Autodesk Inventor part; units mm, degrees
ref_plane "YZ Plane" through (0, 0, 0) normal (1, 0, 0) x (0, 1, 0)
ref_plane "XZ Plane" through (0, 0, 0) normal (0, 1, 0) x (-1, 0, 0)
ref_plane "XY Plane" through (0, 0, 0) normal (0, 0, 1) x (1, 0, 0)
sketch "Sketch1" plane through (0, 0, 0) normal (0, 1, 0) x (-1, 0, 0)
  line L0 (0, 0) -> (29.7942, 0)
  line L1 (29.7942, 0) -> (29.7942, -38.1)
  line L2 (29.7942, -38.1) -> (0, -38.1)
  line L3 (0, -38.1) -> (0, 0)
  circle A0 centre (21.844, -9.525) radius 1.905
  circle A1 centre (8.255, -29.845) radius 1.905
  dimension "d0" = 29.7942
  dimension "d1" = 38.1
  dimension "d2" = 3.81
  dimension "d3" = 3.81
  dimension "d4" = 7.9502
  dimension "d5" = 9.525
  dimension "d6" = 8.255
  dimension "d7" = 8.255
extrude "Extrusion1" add sketch "Sketch1" along normal blind 3.175
sketch "Sketch2" plane through (-29.7942, 0, 0) normal (0, 0, 1) x (1, 0, 0)
  line L0 (29.7942, 0) -> (0, 0)
  line L1 (0, 0) -> (29.7942, 0)
  line L2 (29.7942, 0) -> (29.7942, -177.8)
  line L3 (29.7942, -177.8) -> (0, -177.8)
  line L4 (0, -113.5257) -> (0, 0)
  circle A0 centre (6.9723, -175.3108) radius 1.8034
  circle A1 centre (-16.2433, -164.7952) radius 1.8034
  line L5 (0, -177.8) -> (-18.7325, -177.8)
  line L6 (-18.7325, -177.8) -> (-18.7325, -158.75)
  line L7 (-18.7325, -158.75) -> (0, -113.5257)
  dimension "d11" = 177.8
  dimension "d12" = 3.6068
  dimension "d13" = 3.6068
  dimension "d15" = 13.0048
  dimension "d16" = 2.4892
  dimension "d22" = 157.5
  dimension "d24" = 19.05
  dimension "d25" = 48.5267
  dimension "d26" = 29.7942
  dimension "d27" = 2.4892
  dimension "d28" = 25.7048
extrude "Extrusion2" add sketch "Sketch2" against normal blind 3.81
sketch "Sketch3" plane through (0, 3.175, 0) normal (1, 0, 0) x (0, 0, -1)
  line L0 (3.81, -3.175) -> (3.81, -180.975)
  line L1 (38.1, -3.175) -> (3.81, -180.975)
  line L2 (38.1, -3.175) -> (3.81, -3.175)
  point P0 (0, -3.175)
extrude "Extrusion3" add sketch "Sketch3" against normal blind 3.175
properties part number "LimitSwitchBottomV3"
Here's how the part is built. I have some questions about the finished solid (model axes, mm). A direction names the side the tool comes from. Round coordinates to 2 decimals unless told otherwise and drop trailing zeros. Loops run counter-clockwise (first coordinate to the right, second up) from the corner with the lowest first, then second, coordinate; pieces in that order, holes last. Notation, with made-up numbers: (56, 53.25) -> (73, 53.25) arc R23 cw to (73, 88.25) -> close; hole circle Ø5 at (-5.5, 19.25). An arc over 180 degrees is marked (long way). Write each question's results on one line, items separated by ' | '.
(1) For P1, Ø13.5, axis at x = -20, z = -19.5, coming from the -Y side; P2, Ø2, axis at x = -22.82, y = -175.31, coming from the +Z side; P3, Ø10.5, axis at y = -46.5, z = -22, coming from the -X side (3 decimals), each with a flat end and sliding along its axis, tell me the tip position at first contact or that it passes through.
Worked answers:
P1: y = 0 | P2: through | P3: x = -3.175
(2) If I drill on L1, parallel to X at y = -140.5, z = -10 (3 decimals); L2, parallel to Y at x = -11, z = -5.5 (3 decimals); L3, parallel to Z at x = -16.5, y = -27.5, over which ranges is the centre line in solid material (lowest first)?
Worked answers:
L1: -3.175 to 0 | L2: 0 to 3.175 | L3: -3.81 to 0
(3) We'd pull the mould along X, two halves only. Please class faces 1 (the face through (-3.175, -68, -17)), 2 (the face through (-16, 0, -21)), 3 (the face through (-23.057, -173.523, -1.878)), 4 (the face through (-23.66, 1.57, -10.1)): released by +X, released by -X, zero draft, split by the parting line, or undercut.
Worked answers:
face 1: released by -X | face 2: zero draft | face 3: undercut | face 4: undercut
(4) If we section it at C-C, the plane x = -37: List the corners of the cut face in (y, z) for me, then the cut area to 3 significant figures.
Worked answers:
outline: (-177.8, -3.81) -> (-130.92, -3.81) -> (-130.92, 0) -> (-177.8, 0) -> close | area: 179 mm2
(5) If we section it at A-A, the plane y = -80.5: List the corners of the cut face in (x, z) for me (3 decimals).
Worked answers:
outline: (-29.794, -3.81) -> (-3.175, -3.81) -> (-3.175, -22.575) -> (0, -22.575) -> (0, 0) -> (-29.794, 0) -> close
(6) For faces 5 (the face through (-15, 3.175, -19)), 6 (the face through (-29.794, -42, -3)), 7 (the face through (-21, -107, -3.81)), which set-ups out of +Z, -Z, +X, -X, +Y, -Y let a thin tool reach every point of the face, with its end or its side?
Worked answers:
face 5: +Z, -Z, +X, -X, +Y | face 6: +Z, -Z, -X, +Y | face 7: -Z, -X, -Y
(7) If we section it at B-B, the plane x = -27: List the corners of the cut face in (y, z) for me (3 decimals).
Worked answers:
outline: (-177.8, -3.81) -> (0, -3.81) -> (0, -38.1) -> (3.175, -38.1) -> (3.175, 0) -> (-177.8, 0) -> close
